Design review of the part shown in the three views and the two pictorial views. Dimensions are in mm from the part's minimum x, y and z. Coordinates: 2 decimals unless noted, no trailing zeros. Loops run counter-clockwise (first coordinate to the right, second up) from the corner with the lowest first, then second, coordinate; pieces in that order, holes last. Notation, with made-up numbers: (-9.75, 72) -> (46.25, 72) arc R18 ccw to (46.25, 87) -> close; hole circle Ø5 at (81, 66.5). An arc over 180 degrees is marked (long way). Use a Markdown table: item, result. Add a question column.
Q1. Clearance check with flat-ended pins moving along their axes: pin 1 Ø5 at (x, z) = (29.5, 162) entering from -Y (1 decimal); pin 2 Ø6 at (x, z) = (15, 201) entering from +Y; pin 3 Ø3 at (x, z) = (20.64, 85) entering from +Y (3 decimals); pin 4 Ø4 at (y, z) = (8.5, 82.5) entering from -X. State where each tip first meets the part, or that it passes through.
Q2. Take a section at B-B on y = 30.5. Write out the cut boundary in (x, z) (1 decimal).
Q3. Take a section at A-A on z = 215. Write out the cut boundary in (x, y) (1 decimal).
Q4. Draft analysis for pull direction Y (two halves, no side actions). For the marked faces 1 and 2, state which applies: pulls with the +Y half, pulls with the -Y half, needs draft (parallel to the pull), parting line crosses it, or undercut.
Q5. For probe 1 along Y at (x, z) = (22, 146) (1 decimal); probe 2 along Y at (x, z) = (36, 84) (1 decimal); probe 3 along X at (y, z) = (33, 191.5) (1 decimal), list the stretches that pass through material, from the lowest coordinate up.
Q6. Take a section at C-C on z = 118.5. Write out the cut boundary in (x, y) (1 decimal).
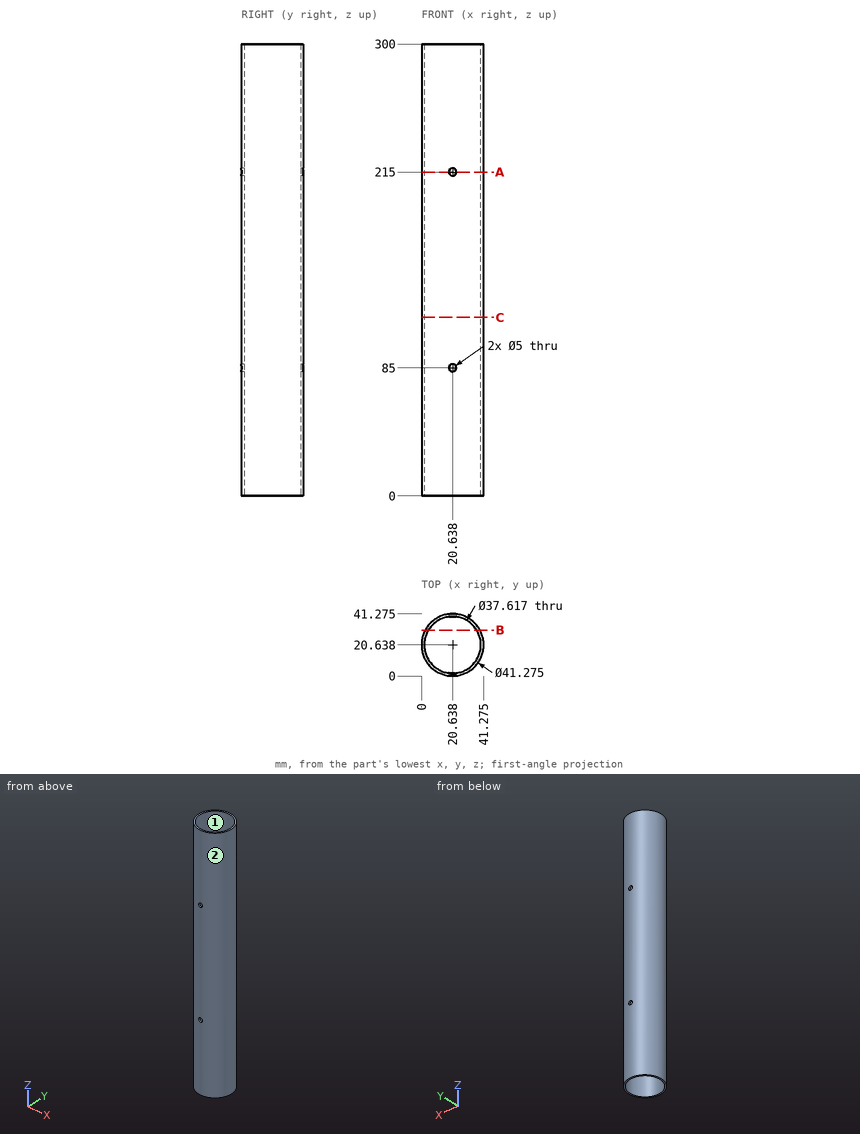
Answer list:
| question | item | result |
|---|---|---|
| 1 | pin 1 | y = 1 |
| 1 | pin 2 | y = 41.11 |
| 1 | pin 3 | through |
| 1 | pin 4 | x = 2.66 |
| 2 | outline | (2.5, 0) -> (4.6, 0) -> (4.6, 300) -> (2.5, 300) -> close; (36.7, 0) -> (38.8, 0) -> (38.8, 300) -> (36.7, 300) -> close |
| 3 | outline | (18.1, 0.2) -> (18.1, 2) arc R18.8 cw to (18.1, 39.3) -> (18.1, 41.1) arc R20.6 ccw to start; (23.1, 0.2) arc R20.6 ccw to (23.1, 41.1) -> (23.1, 39.3) arc R18.8 cw to (23.1, 2) -> close |
| 4 | face 1 | undercut |
| 4 | face 2 | parting line crosses it |
| 5 | probe 1 | 0 to 1.9, 39.4 to 41.2 |
| 5 | probe 2 | 6.9 to 9.8, 31.5 to 34.4 |
| 5 | probe 3 | 4.1 to 6.5, 34.8 to 37.2 |
| 6 | outline | circle Ø41.3 at (20.6, 20.6); hole circle Ø37.6 at (20.6, 20.6) |
